Geometry check sheet. Reference: the model listing, model coordinates, mm. A direction names the side the tool comes from. Give positions to 0.01 mm unless a question says otherwise; leave off trailing zeros. Write each loop counter-clockwise with the first axis right and the second up, starting at its lowest first coordinate (ties: lowest second). Pieces come first, ordered by that corner, then holes. Notation, with made-up numbers: (17.25, 40.25) - (51.25, 40.25) arc R31 ccw to (51.25, 66.25) - close; hole circle Ø4 at (24, 10.5). An arc over 180 degrees is marked (long way). Use a Markdown table: item, result.
Autodesk Inventor part; units mm, degrees
ref_plane "Arbeitsebene1" through (-33.5, 0, 0) normal (-1, 0, 0) x (0, 0, 1)
ref_plane "YZ Plane" through (0, 0, 0) normal (1, 0, 0) x (0, 1, 0)
ref_plane "XZ Plane" through (0, 0, 0) normal (0, 1, 0) x (-1, 0, 0)
sketch "Skizze1" plane through (0, 0, 0) normal (0, 1, 0) x (-1, 0, 0)
  line L0 (0, 0) -> (67, 0)
  line L1 (67, 0) -> (67, 9.1)
  line L2 (67, 9.1) -> (0, 9.1)
  line L3 (0, 9.1) -> (0, 0)
  line L4 (61, 9.1) -> (64, 9.1)
  line L5 (64, 9.1) -> (64, 8.75)
  line L6 (64, 8.75) -> (61, 8.75)
  line L7 (61, 8.75) -> (61, 9.1)
  line L8 (80.4, 0) -> (-13.4, 0)
  dimension "d0" = 67
  dimension "d1" = 9.1
  dimension "d2" = 3
  dimension "d3" = 3
  dimension "d4" = 0.35
revolve "Umdrehung1" add sketch "Skizze1" angle 360 about axis through (-10, 0, 0) along (1, 0, 0) contours L3 L2 L7 L6 L5 L1 L0
ref_plane "Arbeitsebene1" through (-33.5, 0, 0) normal (-1, 0, 0) x (0, 0, 1)
fillet "Rundung1" radius 2 4 edges at (-64, 0, -9.1) (-64, 0, -8.75) (-61, 0, -8.75) (-61, 0, -9.1)
fillet "Rundung2" radius 1 2 edges at (-67, 0, -9.1) (0, 0, -9.1)
sketch "Skizze2" plane through (-67, 0, 0) normal (-1, 0, 0) x (0, 0, 1)
  circle A0 centre (0, 0) radius 8.1
  circle A1 centre (0, 0) radius 6.5
  dimension "d8" = 13
extrude "Extrusion1" cut sketch "Skizze2" against normal blind 0.2 contours A1
mirror "Spiegeln1" about plane through (-33.5, 0, 0) normal (-1, 0, 0) of "Extrusion1"
sketch "Skizze3" plane through (-66.8, 0, 0) normal (-1, 0, 0) x (0, 0, 1)
  circle A0 centre (0, 0) radius 6.5
  circle A1 centre (0, 0) radius 2.85
  dimension "d11" = 5.7
extrude "Extrusion2" add sketch "Skizze3" along normal blind 1 contours A1
fillet "Rundung3" radius 0.5 1 edges at (-67.8, 0, -2.85)
sketch "Skizze4" plane through (-0.2, 0, 0) normal (1, 0, 0) x (0, 0, -1)
  circle A0 centre (0, 0) radius 6.5
  circle A1 centre (0, 0) radius 5.5
  dimension "d15" = 1
extrude "Extrusion3" add sketch "Skizze4" along normal blind 0.2 contours A1
fillet "Rundung4" radius 0.5 1 edges at (0, 0, 5.5)
properties part number "accu_18500"
1) Section check A-A on x = -30. Record the boundary of the cut face in (y, z).
Working result:
| item | result |
|---|---|
| outline | circle Ø18.2 at (0, 0) |
2) Material ranges on L1, parallel to Y at x = -66.85, z = 0; L2, parallel to Y at x = -0.1, z = 0; L3, parallel to X at y = 5, z = -3.75, recorded low to high. Write a range as from..to.
Working result:
| item | result |
|---|---|
| L1 | y = -8.63..-6.5, -2.85..2.85, 6.5..8.63 |
| L2 | y = -8.54..-6.5, -5.4..5.4, 6.5..8.54 |
| L3 | x = -66.8..-0.2 |
3) Set-up check for faces 5 (the flat face through (0, -7, 0)), 6 (the cylindrical face through (-67.046, 1.734, -2.262)), 7 (the cylindrical face through (-62.803, 5.324, -6.944)): record each of +Z, -Z, +X, -X, +Y, -Y from which the full face is reachable in a straight line by a thin tool's end or side.
Working result:
| item | result |
|---|---|
| face 5 | +Z, -Z, +X, +Y, -Y |
| face 6 | -X |
| face 7 | none |
4) Mould release check, pull along Z, two halves, no side actions. Record for faces 1 (the cylindrical face through (-65.559, 8.884, -1.973)), 2 (the flat face through (-66.8, -1, 3)), 3 (the flat face through (-67.8, 0, 0)), 4 (the flat face through (-0.2, 3, 5)): pulls with the +Z half, pulls with the -Z half, needs draft (parallel to the pull), parting line crosses it, or undercut.
Working result:
| item | result |
|---|---|
| face 1 | parting line crosses it |
| face 2 | undercut |
| face 3 | needs draft |
| face 4 | undercut |
5) Depth check by flat-ended pin: P1, Ø6, axis at x = -10.5, y = -5.5, coming from the -Z side; P2, Ø10, axis at x = -12, y = -4.5, coming from the +Z side; P3, Ø1, axis at x = -15, z = 4, coming from the +Y side. Enter the tip coordinate at first touch or a pass-through.
Working result:
| item | result |
|---|---|
| P1 | stops at z = -8.75 |
| P2 | stops at z = 9.1 |
| P3 | stops at y = 8.4 |
